```python
from build123d import *

# Parameters (mm, degrees)
SKETCH1_W            = 800
SKETCH1_H            = 363
BOSS_EXTRUDE1_DEPTH  = 30
SKETCH2_R            = 12.5
CUT_EXTRUDE1_DEPTH   = 30
LPATTERN1_COUNT      = 3
LPATTERN1_PITCH      = 149
LPATTERN1_COUNT_DIR2 = 2
LPATTERN1_PITCH_DIR2 = 735
SKETCH3_R            = 6
CUT_EXTRUDE2_DEPTH   = 20
LPATTERN2_COUNT      = 5
LPATTERN2_PITCH      = 82
SKETCH4_R            = 5
CUT_EXTRUDE3_DEPTH   = 18
LPATTERN3_COUNT      = 10
LPATTERN3_PITCH      = 68.33
FILLET1_R            = 3


with BuildPart() as part:
    # Sketch1 → Boss-Extrude1 (new body)
    with BuildSketch(Plane.XY):
        with Locations((400, 181.5)):
            Rectangle(SKETCH1_W, SKETCH1_H)
    extrude(amount=BOSS_EXTRUDE1_DEPTH)

    # Sketch2 → Cut-Extrude1 (cut)
    with BuildSketch(Plane.XY.offset(30)):
        with Locations((32.5, 32.5)):
            Circle(SKETCH2_R)
    cut_extrude1 = extrude(amount=-CUT_EXTRUDE1_DEPTH, mode=Mode.SUBTRACT)

    # LPattern1: Cut-Extrude1 3 × 2
    with Locations(*[(j * LPATTERN1_PITCH_DIR2, i * LPATTERN1_PITCH, 0) for i in range(LPATTERN1_COUNT) for j in range(LPATTERN1_COUNT_DIR2) if (i, j) != (0, 0)]):
        add(cut_extrude1, mode=Mode.SUBTRACT)

    # Sketch3 → Cut-Extrude2 (cut)
    with BuildSketch(Plane.XY.offset(30)):
        with Locations((236, 150)):
            Circle(SKETCH3_R)
    cut_extrude2 = extrude(amount=-CUT_EXTRUDE2_DEPTH, mode=Mode.SUBTRACT)

    # LPattern2: Cut-Extrude2 ×5
    with Locations(*[(i * LPATTERN2_PITCH, 0, 0) for i in range(1, LPATTERN2_COUNT)]):
        add(cut_extrude2, mode=Mode.SUBTRACT)

    # Sketch4 → Cut-Extrude3 (cut)
    with BuildSketch(Plane.XZ):
        with Locations((92.53, 10)):
            Circle(SKETCH4_R)
    cut_extrude3 = extrude(amount=-CUT_EXTRUDE3_DEPTH, mode=Mode.SUBTRACT)

    # LPattern3: Cut-Extrude3 ×10
    with Locations(*[(i * LPATTERN3_PITCH, 0, 0) for i in range(1, LPATTERN3_COUNT)]):
        add(cut_extrude3, mode=Mode.SUBTRACT)

    # Fillet1
    fillet1_edges = [part.edges().sort_by_distance(p)[0] for p in [
        (800, 181.5, 30),
        (400, 363, 30),
        (0, 181.5, 30),
        (400, 363, 0),
        (800, 181.5, 0),
        (400, 0, 0),
        (0, 181.5, 0),
        (0, 363, 15),
        (800, 363, 15),
        (800, 0, 15),
        (0, 0, 15),
        (400, 0, 30),
    ]]
    fillet(fillet1_edges, radius=FILLET1_R)


solid = part.part
```
CAD build for the part. Positions are in the model's coordinates, mm. Round coordinates to 2 decimals unless told otherwise and drop trailing zeros. Loops run counter-clockwise (first coordinate to the right, second up) from the corner with the lowest first, then second, coordinate; pieces in that order, holes last. Notation, with made-up numbers: (30, 79) - (37, 79) arc R17 ccw to (37, 102) - close; hole circle Ø1 at (-22, 34). An arc over 180 degrees is marked (long way). Return JSON: item names as keys, results as strings. Group by question number.
Q1. Band-saw the part on B-B on x = 32.5. Give the cut face in (y, z), plus the area to 3 significant figures.
Q2. Flat gauge pins, fed straight in: pin 1 Ø3 at (x, z) = (436, 10) entering from -Y; pin 2 Ø9.5 at (x, y) = (318, 150) entering from +Z. Where does each tip first touch, or does it go through?
Q3. Band-saw the part on A-A on y = 330.5. Give the cut face in (x, z).
Q4. Two-plate mould, pull along Y, no slides. Class faces 1 (the face through (758.29, 189.95, 15.21)), 2 (the face through (29.79, 318.297, 15.21)), 3 (the face through (394, 0, 15)), 4 (the face through (394, 363, 15)): +Y half, -Y half, draft (parallel to the pull), parting line (faces both ways), or undercut.
Q5. Drill centre lines: line 1 along Y through (x, z) = (767.5, 10.5); line 2 along Z through (x, y) = (502, 13); line 3 along Y through (x, z) = (482, 16.5). Where is each one in solid material? Low to high. Write a range as [from, to].
Solutions:
{
 "1": {"outline": "(0, 3) arc R3 ccw to (3, 0) - (20, 0) - (20, 30) - (3, 30) arc R3 ccw to (0, 27) - close; (45, 0) - (169, 0) - (169, 30) - (45, 30) - close; (194, 0) - (318, 0) - (318, 30) - (194, 30) - close; (343, 0) - (360, 0) arc R3 ccw to (363, 3) - (363, 27) arc R3 ccw to (360, 30) - (343, 30) - close", "area": "8,630 mm^2"},
 "2": {"pin 1": "stops at y = 18", "pin 2": "stops at z = 10"},
 "3": {"outline": "(0, 3) arc R3 ccw to (3, 0) - (20, 0) - (20, 30) - (3, 30) arc R3 ccw to (0, 27) - close; (45, 0) - (755, 0) - (755, 30) - (45, 30) - close; (780, 0) - (797, 0) arc R3 ccw to (800, 3) - (800, 27) arc R3 ccw to (797, 30) - (780, 30) - close"},
 "4": {"face 1": "undercut", "face 2": "undercut", "face 3": "-Y half", "face 4": "+Y half"},
 "5": {"line 1": "y = [0, 20], [45, 169], [194, 318], [343, 363]", "line 2": "z = [0, 5.03], [14.97, 30]", "line 3": "y = [0, 144], [156, 363]"}
}
